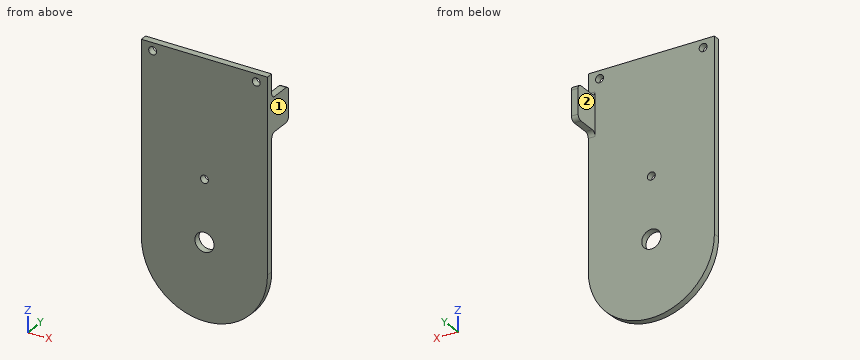
from build123d import *

# Parameters (mm, degrees)
SKETCH1_R           = 1.75
SKETCH1_R_2         = 4.25
BOSS_EXTRUDE1_DEPTH = 3
SKETCH2_W           = 3
SKETCH2_H           = 15.115775603
BOSS_EXTRUDE2_DEPTH = 12
FILLET1_R           = 2


with BuildPart() as part:
    # Sketch1 → Boss-Extrude1 (new body)
    with BuildSketch(Plane(origin=(0, 0, 0), x_dir=(1, 0, 0), z_dir=(0, 1, 0))):
        with BuildLine():
            Line((0, 0), (0, -85))
            Line((0, -85), (56, -85))
            Line((56, -85), (56, 6.6e-08))
            ThreePointArc((56, 6.6e-08), (27.999999967, 28.000000033), (0, 0))
        make_face()
        with Locations((5, -81.5)):
            Circle(SKETCH1_R, mode=Mode.SUBTRACT)
        with Locations((51, -81.5)):
            Circle(SKETCH1_R, mode=Mode.SUBTRACT)
        with Locations((28, -33)):
            Circle(SKETCH1_R, mode=Mode.SUBTRACT)
        with Locations((28, -5.94)):
            Circle(SKETCH1_R_2, mode=Mode.SUBTRACT)
    extrude(amount=BOSS_EXTRUDE1_DEPTH)

    # Sketch2 → Boss-Extrude2 (add)
    with BuildSketch(Plane(origin=(0, 3, 0), x_dir=(1, 0, 0), z_dir=(0, 1, 0))):
        with Locations((54.5, -66.844146369)):
            Rectangle(SKETCH2_W, SKETCH2_H)
    extrude(amount=BOSS_EXTRUDE2_DEPTH)

    # Fillet1
    fillet1_edges = [part.edges().sort_by_distance(p)[0] for p in [
        (54.5, 3, 59.286258567),
        (54.5, 3, 74.40203417),
        (54.5, 15, 59.286258567),
        (54.5, 15, 74.40203417),
    ]]
    fillet(fillet1_edges, radius=FILLET1_R)


solid = part.part
Source: CAD feature listing. Evaluate the final solid. Frame: model axes, mm. Face numbers are marked on the shaded views. A direction names the side the tool comes from. Give positions to 0.01 mm unless a question says otherwise; leave off trailing zeros. Write each loop counter-clockwise with the first axis right and the second up, starting at its lowest first coordinate (ties: lowest second). Pieces come first, ordered by that corner, then holes. Notation, with made-up numbers: M 70.25,60 L 74.25,60 A28 cw 74.25,98 Z; hole C -7,8 d9. An arc over 180 degrees is marked long. Return JSON: item names as keys, results as strings. Group by question number.
1) Set-up query: the marked faces 1 and 2. Return all of +Z, -Z, +X, -X, +Y, -Y with unobstructed straight access to the full face (end or side cutting, diameter ignored); none if empty.
2) First-contact query: pin 1 Ø17 at (x, z) = (14.5, 46) entering from +Y; pin 2 Ø1.5 at (x, y) = (54.5, 8) entering from +Z; pin 3 Ø1.5 at (x, y) = (25.5, 3.5) entering from -Z. Flat tips, straight axial feed; report the tip coordinate or a pass-through.
3) Cut plane A-A, the plane x = 28. Output: boundary loops of the cut face in (y, z), then the cut area to 3 significant figures.
4) Cut plane D-D, the plane z = 81.5. Output: boundary loops of the cut face in (x, y), then the cut area to 3 significant figures.
5) Cut plane C-C, the plane y = 1.5. Output: boundary loops of the cut face in (x, z), then the cut area to 3 significant figures.
6) Ray query, L1, parallel to X at y = 1.7, z = 81.5; L2, parallel to Z at x = 28, y = 1.85; L3, parallel to Y at x = 5, z = 2.5. Return the intervals inside material, ascending.
7) Cut plane B-B, the plane z = 33. Output: boundary loops of the cut face in (x, y), then the cut area to 4 significant figures.
Data:
{
 "1": {"face 1": "+Z, -Z, +X, +Y, -Y", "face 2": "+Z, -Z, -X, +Y"},
 "2": {"pin 1": "stops at y = 3", "pin 2": "stops at z = 74.4", "pin 3": "stops at z = -27.93"},
 "3": {"outline": "M 0,-28 L 3,-28 L 3,1.69 L 0,1.69 Z; M 0,10.19 L 3,10.19 L 3,31.25 L 0,31.25 Z; M 0,34.75 L 3,34.75 L 3,85 L 0,85 Z", "area": "303 mm²"},
 "4": {"outline": "M 0,0 L 3.25,0 L 3.25,3 L 0,3 Z; M 6.75,0 L 49.25,0 L 49.25,3 L 6.75,3 Z; M 52.75,0 L 56,0 L 56,3 L 52.75,3 Z", "area": "147 mm²"},
 "5": {"outline": "M 0,0 A28 ccw 56,0 L 56,85 L 0,85 Z; hole C 5,81.5 d3.5; hole C 28,5.94 d8.5; hole C 28,33 d3.5; hole C 51,81.5 d3.5", "area": "5,910 mm²"},
 "6": {"L1": "x = 0 to 3.25, 6.75 to 49.25, 52.75 to 56", "L2": "z = -28 to 1.69, 10.19 to 31.25, 34.75 to 85", "L3": "y = 0 to 3"},
 "7": {"outline": "M 0,0 L 26.25,0 L 26.25,3 L 0,3 Z; M 29.75,0 L 56,0 L 56,3 L 29.75,3 Z", "area": "157.5 mm²"}
}
